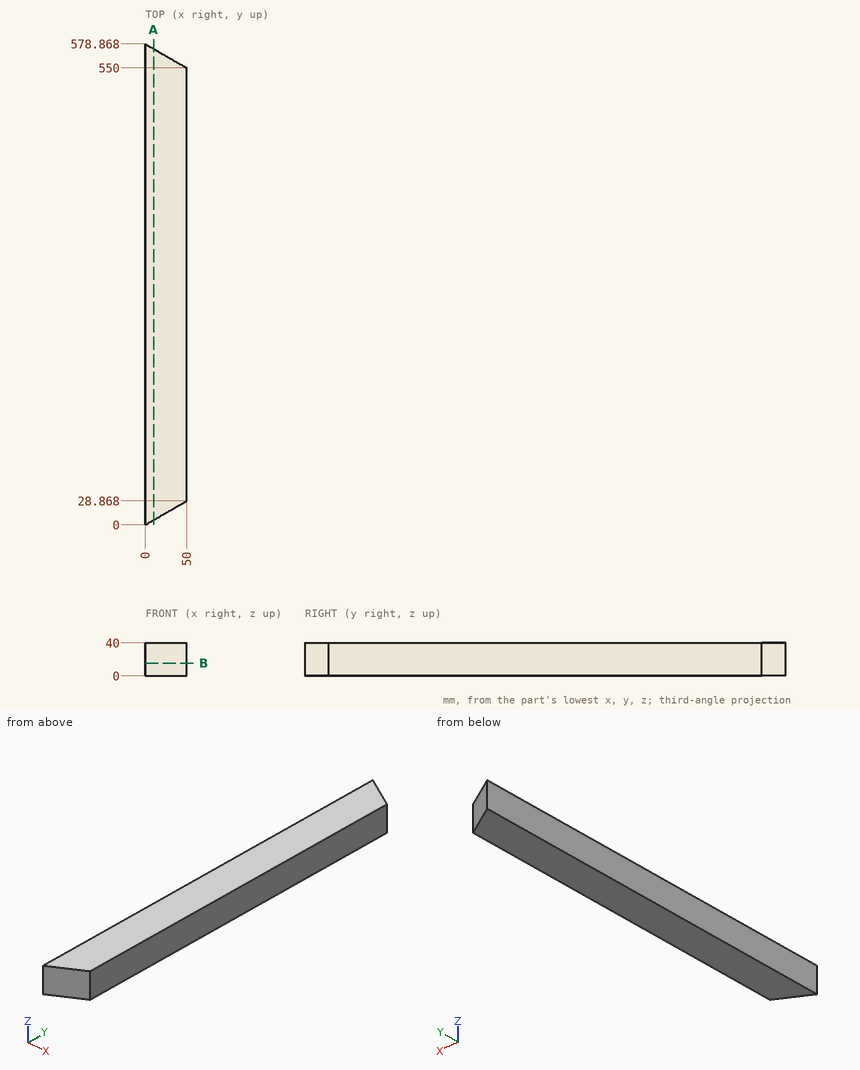
Design review of the part shown in the three views and the two pictorial views. Dimensions are in mm from the part's minimum x, y and z. Coordinates: 2 decimals unless noted, no trailing zeros. Loops run counter-clockwise (first coordinate to the right, second up) from the corner with the lowest first, then second, coordinate; pieces in that order, holes last. Notation, with made-up numbers: (-1.75, 3.5) - (42.25, 3.5) arc R28 ccw to (42.25, 37.5) - close; hole circle Ø3 at (-17.75, 9.5). An arc over 180 degrees is marked (long way). Use a Markdown table: item, result. Add a question column.
Item 1: We need section B-B (z = 15.5). Give the boundary of the cut face in (x, y), and give its area (3 significant figures).
Item 2: Insertion check: pin 1 Ø6 at (x, y) = (8, 489.5) entering from -Z; pin 2 Ø1 at (x, z) = (12, 8) entering from -Y; pin 3 Ø2 at (x, z) = (42, 21.5) entering from -Y; pin 4 Ø8 at (x, z) = (18.5, 10) entering from -Y. Each pin has a flat end and moves straight along its axis. Give the tip position at first contact, or say it passes through.
Item 3: We need section A-A (x = 10). Give the boundary of the cut face in (y, z), and give its area (3 significant figures).
Item 4: For line 1 (Y direction, x = 19.5, z = 35); line 2 (Y direction, x = 41, z = 22) (1 decimal), list the stretches that pass through material, from the lowest coordinate up.
Results list:
| question | item | result |
|---|---|---|
| 1 | outline | (0, 0) - (50, 28.87) - (50, 550) - (0, 578.87) - close |
| 1 | area | 27,500 mm^2 |
| 2 | pin 1 | stops at z = 0 |
| 2 | pin 2 | stops at y = 6.64 |
| 2 | pin 3 | stops at y = 23.67 |
| 2 | pin 4 | stops at y = 8.37 |
| 3 | outline | (5.77, 0) - (573.09, 0) - (573.09, 40) - (5.77, 40) - close |
| 3 | area | 22,700 mm^2 |
| 4 | line 1 | y = 11.26 to 567.61 |
| 4 | line 2 | y = 23.7 to 555.2 |
